Input: dimensioned drawing with shaded views. Units: mm. Origin: part minimum x, y, z. Round coordinates to 2 decimals unless told otherwise and drop trailing zeros. Write each loop counter-clockwise with the first axis right and the second up, starting at its lowest first coordinate (ties: lowest second). Pieces come first, ordered by that corner, then holes. Notation, with made-up numbers: (70, 67.5) - (101, 67.5) arc R6 cw to (101, 75.5) - close; hole circle Ø8 at (-19, -19.5). An arc over 180 degrees is marked (long way). Use one line per item in the form item = value.
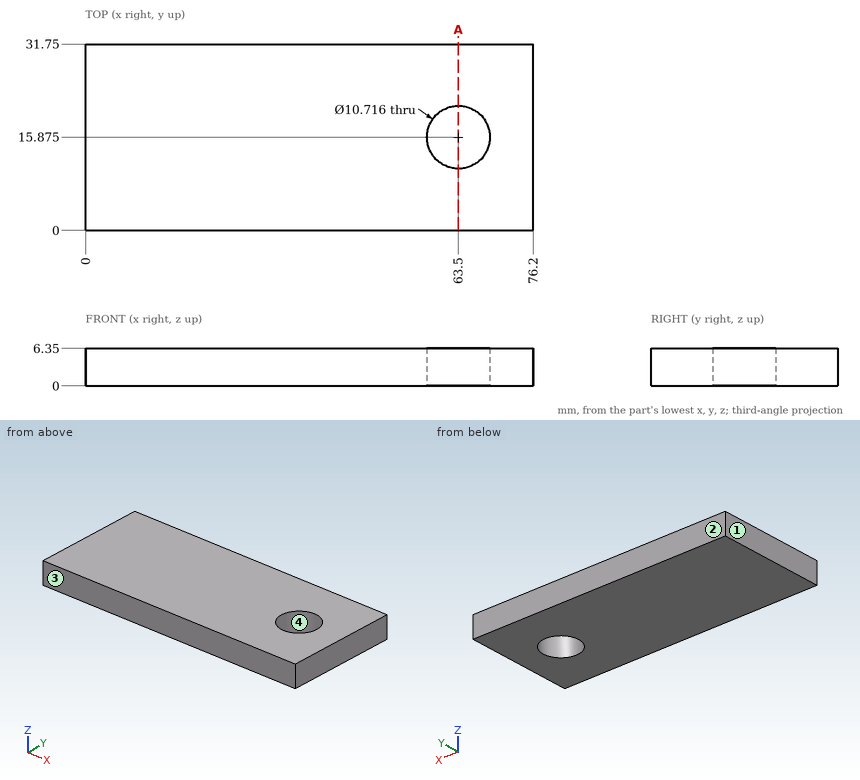
(1) Cut plane A-A on x = 63.5. Output: boundary loops of the cut face in (y, z), then the cut area to 3 significant figures.
Derived:
outline = (0, 0) - (10.52, 0) - (10.52, 6.35) - (0, 6.35) - close; (21.23, 0) - (31.75, 0) - (31.75, 6.35) - (21.23, 6.35) - close
area = 134 mm^2
(2) Material intervals for L1, parallel to Y at x = 63.5, z = 1.5; L2, parallel to X at y = 16, z = 5.25; L3, parallel to X at y = 15, z = 4, sorted ascending.
Derived:
L1 = 0 to 10.52, 21.23 to 31.75
L2 = 0 to 58.14, 68.86 to 76.2
L3 = 0 to 58.21, 68.79 to 76.2
(3) Draft query along Y for the marked faces 1, 2, 3 and 4. Return one class per face: released by +Y, released by -Y, zero draft, split by the parting line, or undercut.
Derived:
face_1 = zero draft
face_2 = released by +Y
face_3 = released by -Y
face_4 = undercut
